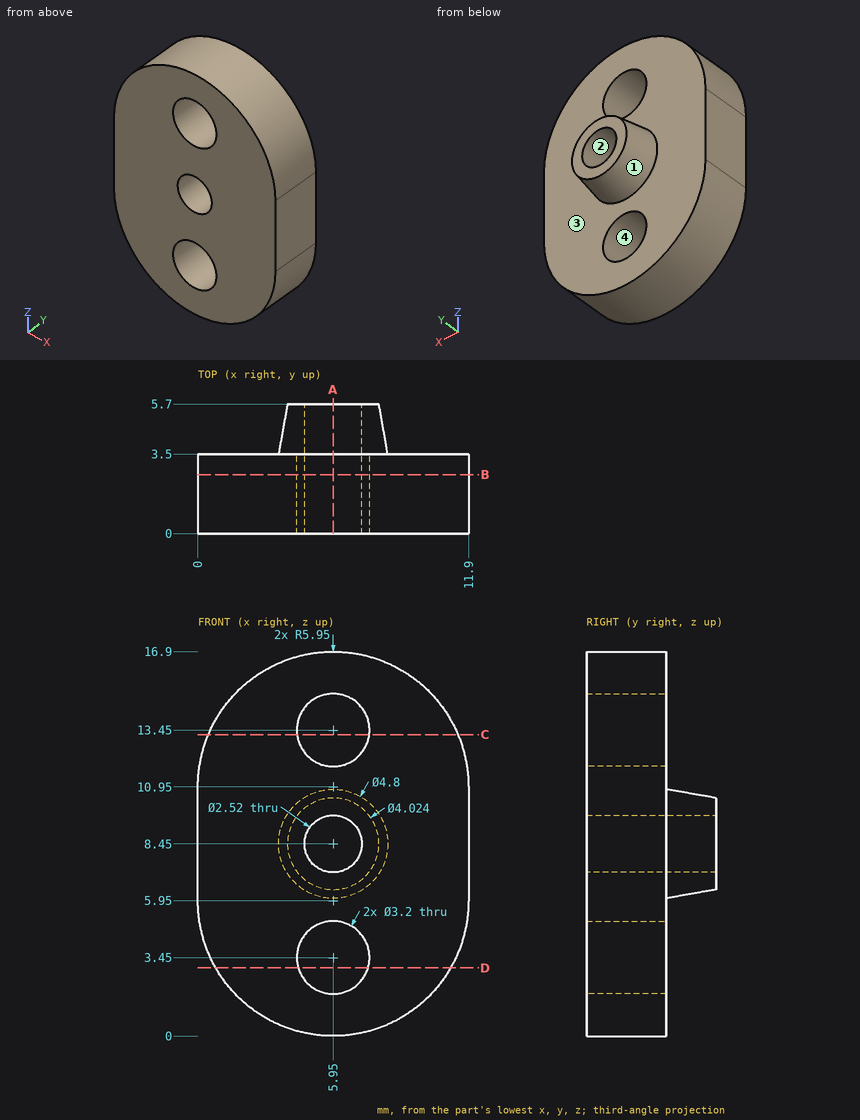
Drawing for the job (mm, zero at the part's lowest x, y, z). Coordinates: 2 decimals unless noted, no trailing zeros. Order: outer loops, then holes, each group sorted by start corner. A loop starts at its lowest first (then second) coordinate and runs counter-clockwise, first axis right, second up. Notation, with made-up numbers: (51, -14) - (86, -14) arc R13 cw to (86, 1) - close; hole circle Ø6 at (-20.75, 70.5). An arc over 180 degrees is marked (long way). Use a Markdown table: item, result. Add a question column.
(1) Pull direction X, two halves, no side cores. Call the marked faces 1, 2, 3 and 4: +X half, -X half, draft (parallel to the pull), parting line (faces both ways), or undercut.
(2) Saw through at A-A (x = 5.95). Give the cut face in (y, z), then the cut area to 3 significant figures.
(3) Saw through at B-B (y = 2.6). Give the cut face in (x, z), then the cut area to 3 significant figures.
(4) Drill centre lines: line 1 along Z through (x, y) = (5, 2.45); line 2 along Y through (x, z) = (11.25, 7.25); line 3 along X through (y, z) = (4.2, 9.5). Where is each one in solid material? Low to high. Write a range as [from, to].
(5) Saw through at C-C (z = 13.25). Give the cut face in (x, y).
(6) Saw through at D-D (z = 3). Give the cut face in (x, y).
(7) Flat gauge pins, fed straight in: pin 1 (1 mm diameter, centred on x = 10, y = 2.5, fed in from -Z) (1 decimal); pin 2 (1.5 mm diameter, centred on x = 4, y = 0.5, fed in from +Z); pin 3 (5 mm diameter, centred on x = 5.95, z = 3.45, fed in from +Y). Where does each tip first touch, or does it go through?
Solved:
| question | item | result |
|---|---|---|
| 1 | face 1 | parting line |
| 1 | face 2 | undercut |
| 1 | face 3 | draft |
| 1 | face 4 | undercut |
| 2 | outline | (0, 0) - (3.5, 0) - (3.5, 1.85) - (0, 1.85) - close; (0, 5.05) - (3.5, 5.05) - (3.5, 6.05) - (5.7, 6.44) - (5.7, 7.19) - (0, 7.19) - close; (0, 9.71) - (5.7, 9.71) - (5.7, 10.46) - (3.5, 10.85) - (3.5, 11.85) - (0, 11.85) - close; (0, 15.05) - (3.5, 15.05) - (3.5, 16.9) - (0, 16.9) - close |
| 2 | area | 32.1 mm² |
| 3 | outline | (0, 5.95) arc R5.95 ccw to (11.9, 5.95) - (11.9, 10.95) arc R5.95 ccw to (0, 10.95) - close; hole circle Ø3.2 at (5.95, 3.45); hole circle Ø3.2 at (5.95, 13.45); hole circle Ø2.52 at (5.95, 8.45) |
| 3 | area | 150 mm² |
| 4 | line 1 | z = [0.08, 2.16], [4.74, 7.62], [9.28, 12.16], [14.74, 16.82] |
| 4 | line 2 | y = [0, 3.5] |
| 4 | line 3 | x = [3.93, 5.25], [6.65, 7.97] |
| 5 | outline | (0.46, 0) - (4.36, 0) - (4.36, 3.5) - (0.46, 3.5) - close; (7.54, 0) - (11.44, 0) - (11.44, 3.5) - (7.54, 3.5) - close |
| 6 | outline | (0.78, 0) - (4.41, 0) - (4.41, 3.5) - (0.78, 3.5) - close; (7.49, 0) - (11.12, 0) - (11.12, 3.5) - (7.49, 3.5) - close |
| 7 | pin 1 | stops at z = 1.2 |
| 7 | pin 2 | stops at z = 16.78 |
| 7 | pin 3 | stops at y = 3.5 |
